Here's how the part is built. I have some questions about the finished solid (model axes, mm). Face numbers are marked on the shaded views. Coordinates: 2 decimals unless noted, no trailing zeros. Write each loop counter-clockwise with the first axis right and the second up, starting at its lowest first coordinate (ties: lowest second). Pieces come first, ordered by that corner, then holes. Notation, with made-up numbers: (63.25, -29) -> (87.25, -29) arc R27 cw to (87.25, 7) -> close; hole circle Ø9 at (39.5, -39.5). An arc over 180 degrees is marked (long way). Put each result on its own line as item: value.
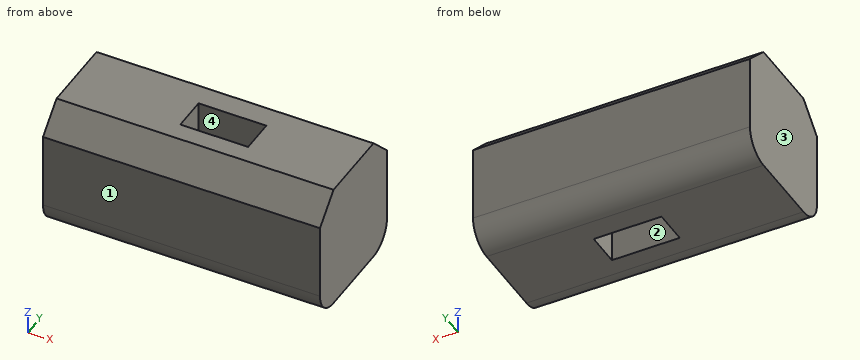
```python
from build123d import *

# Parameters (mm, degrees)
F0_W     = 55.216648
F0_H     = 25.118159
F1_DEPTH = 25.4
F2_W     = 13.522635
F2_H     = 6.827985
F3_DEPTH = 25.4
F4_SIZE  = 5.08
F5_R     = 5.08


with BuildPart() as f1:
    # F0 (on Top) → F1 (new body)
    with BuildSketch(Plane.XY):
        with Locations((6.929148, 1.948819)):
            Rectangle(F0_W, F0_H)
    extrude(amount=F1_DEPTH)

    # F2 (on face) → F3 (cut)
    with BuildSketch(Plane.XY.offset(25.4)):
        with Locations((8.785194, 1.576447)):
            Rectangle(F2_W, F2_H)
    extrude(amount=-F3_DEPTH, mode=Mode.SUBTRACT)

    # F4
    f4_edges = [f1.edges().sort_by_distance(p)[0] for p in [
        (6.929148, 14.507899, 25.4),
        (6.929148, -10.61026, 25.4),
    ]]
    chamfer(f4_edges, length=F4_SIZE)

    # F5
    f5_edges = [f1.edges().sort_by_distance(p)[0] for p in [
        (6.929148, -10.61026, 0),
        (6.929148, 14.507899, 0),
    ]]
    fillet(f5_edges, radius=F5_R)


solid = f1.part
```
Item 1: Imagine slicing it at C-C on x = 4. Write out the boundary of the cut face in (y, z), then the cut area to 3 significant figures.
Output:
outline: (-10.61, 5.08) arc R5.08 ccw to (-5.53, 0) -> (-1.84, 0) -> (-1.84, 25.4) -> (-5.53, 25.4) -> (-10.61, 20.32) -> close; (4.99, 0) -> (9.43, 0) arc R5.08 ccw to (14.51, 5.08) -> (14.51, 20.32) -> (9.43, 25.4) -> (4.99, 25.4) -> close
area: 428 mm²
Item 2: Please list where these lines run through material, in increasing order: line 1 along Y through (x, z) = (12, 7.5); line 2 along X through (y, z) = (3, 23.25); line 3 along Y through (x, z) = (12, 4.25). Write a range as from..to.
Output:
line 1: y = -10.61..-1.84, 4.99..14.51
line 2: x = -20.68..2.02, 15.55..34.54
line 3: y = -10.54..-1.84, 4.99..14.44
Item 3: Imagine slicing it at D-D on y = -6.25. Write out the boundary of the cut face in (x, z).
Output:
outline: (-20.68, 0.05) -> (34.54, 0.05) -> (34.54, 24.68) -> (-20.68, 24.68) -> close
Item 4: Imagine slicing it at A-A on y = 1.5. Write out the boundary of the cut face in (x, z), then the cut area to 3 significant figures.
Output:
outline: (-20.68, 0) -> (2.02, 0) -> (2.02, 25.4) -> (-20.68, 25.4) -> close; (15.55, 0) -> (34.54, 0) -> (34.54, 25.4) -> (15.55, 25.4) -> close
area: 1,060 mm²
Item 5: If we mould it in two halves opening along X, with no side actions, what happens to the marked faces 1, 2, 3 and 4? For each: released by +X, released by -X, zero draft, split by the parting line, or undercut.
Output:
face 1: zero draft
face 2: undercut
face 3: released by -X
face 4: undercut
Item 6: Imagine slicing it at B-B on z = 11.25. Write out the boundary of the cut face in (x, y), then the cut area to 3 significant figures.
Output:
outline: (-20.68, -10.61) -> (34.54, -10.61) -> (34.54, 14.51) -> (-20.68, 14.51) -> close; hole (2.02, -1.84) -> (15.55, -1.84) -> (15.55, 4.99) -> (2.02, 4.99) -> close
area: 1,290 mm²
